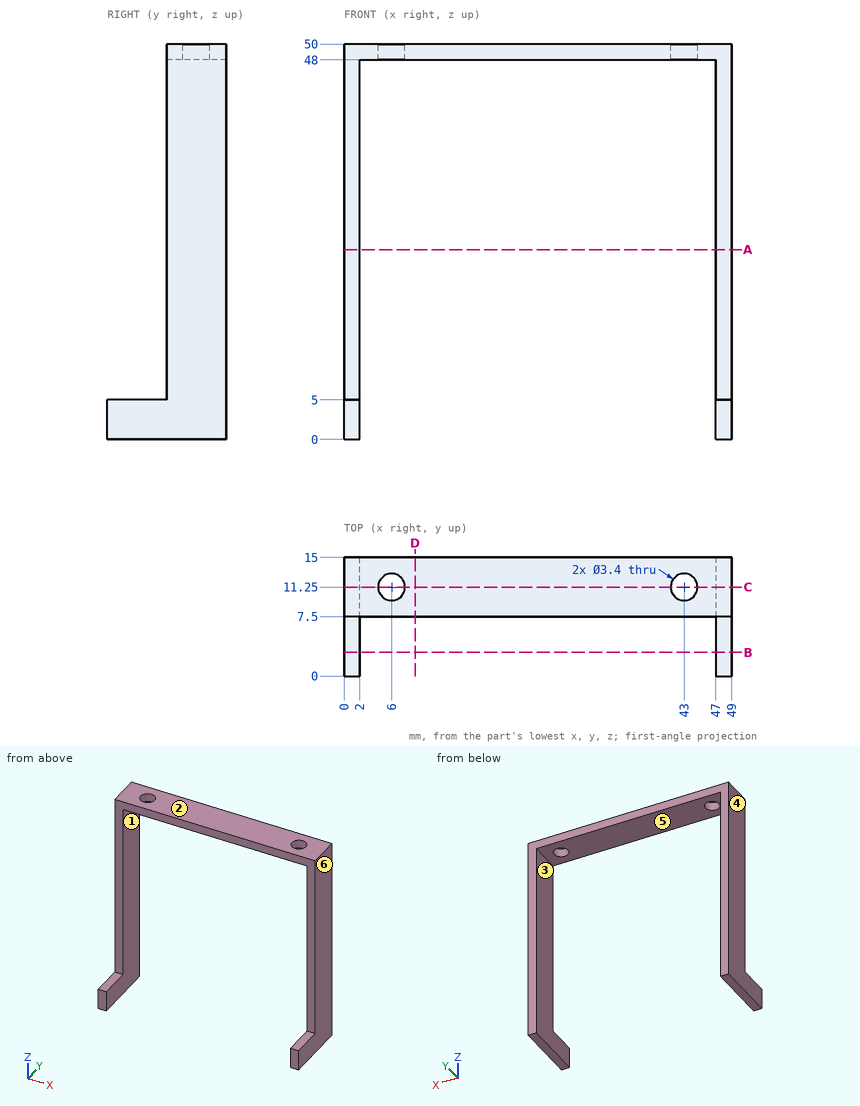
The figure shows three views and two pictorial views of one solid part (mm, origin at its lowest corner). Answer the questions. A direction names the side the tool comes from. Round coordinates to 2 decimals unless told otherwise and drop trailing zeros. Order: outer loops, then holes, each group sorted by start corner. A loop starts at its lowest first (then second) coordinate and runs counter-clockwise, first axis right, second up. Notation, with made-up numbers: (30, 54.25) - (55, 54.25) arc R14 cw to (55, 69.25) - close; hole circle Ø5 at (80, -24.5). An arc over 180 degrees is marked (long way). Write item = value, one per line. Start each with the question number.
1) Section C-C, the plane y = 11.25 is taken. Write down the section's boundary in (x, z).
2) Section A-A, the plane z = 24 is taken. Write down the section's boundary in (x, y).
3) Section D-D, the plane x = 9 is taken. Write down the section's boundary in (y, z).
4) For a pull along X with two mould halves and no side action, classify the marked faces 1, 2, 3 and 4 as released by +X, released by -X, zero draft, split by the parting line, or undercut.
5) Given pin 1 (2.5 mm diameter, centred on x = 43, y = 11.25, fed in from +Z); pin 2 (2 mm diameter, centred on x = 48.5, y = 3, fed in from +Z); pin 3 (4 mm diameter, centred on x = 12, y = 8.5, fed in from -Z), each flat-ended and moving along its own axis, determine where each tip first touches the part or whether it passes through.
6) Straight lines are drawn through the part: L1, parallel to X at y = 11.25, z = 49.25; L2, parallel to X at y = 10, z = 5.5; L3, parallel to Y at x = 43, z = 48.8. For each, find the intervals that lie inside material, in ascending order.
7) For the marked faces 5 and 6, determine the directions among +Z, -Z, +X, -X, +Y, -Y from which every point of the face is accessible in a straight line to the end or side of a thin tool.
8) Section B-B, the plane y = 3 is taken. Write down the section's boundary in (x, z).
Results list:
q1.outline = (0, 0) - (2, 0) - (2, 48) - (4.3, 48) - (4.3, 50) - (0, 50) - close; (7.7, 48) - (41.3, 48) - (41.3, 50) - (7.7, 50) - close; (44.7, 48) - (47, 48) - (47, 0) - (49, 0) - (49, 50) - (44.7, 50) - close
q2.outline = (0, 7.5) - (2, 7.5) - (2, 15) - (0, 15) - close; (47, 7.5) - (49, 7.5) - (49, 15) - (47, 15) - close
q3.outline = (7.5, 48) - (15, 48) - (15, 50) - (7.5, 50) - close
q4.face_1 = undercut
q4.face_2 = zero draft
q4.face_3 = undercut
q4.face_4 = released by -X
q5.pin_1 = through
q5.pin_2 = 5
q5.pin_3 = 48
q6.L1 = 0 to 4.3, 7.7 to 41.3, 44.7 to 49
q6.L2 = 0 to 2, 47 to 49
q6.L3 = 7.5 to 9.55, 12.95 to 15
q7.face_5 = -Z, +Y, -Y
q7.face_6 = +Z, -Z, +X, +Y, -Y
q8.outline = (0, 0) - (2, 0) - (2, 5) - (0, 5) - close; (47, 0) - (49, 0) - (49, 5) - (47, 5) - close
